from build123d import *

# Parameters (mm, degrees)
SKETCH004_W      = 57.0675
SKETCH004_H      = 36.03
EXTRUDE004_DEPTH = 2
SKETCH005_W      = 57.0675
SKETCH005_H      = 36.03
SKETCH005_R      = 3.5
SKETCH005_R_2    = 2
SKETCH005_W_2    = 9
SKETCH005_H_2    = 3.9474
SKETCH005_W_3    = 4.25
SKETCH005_H_3    = 22
EXTRUDE005_DEPTH = 2


with BuildPart() as obj1:
    # Sketch004 → Extrude004 (new body)
    with BuildSketch(Plane.XY.offset(9)):
        with Locations((15.9391, 12.4324)):
            Rectangle(SKETCH004_W, SKETCH004_H)
        Polygon((-11.59465, 29.4474), (43.47285, 29.4474), (43.47285, -4.5826), (-11.59465, -4.5826), (-11.59465, 5.4324), (-10.59465, 5.4324), (-10.59465, 19.4324), (-11.59465, 19.4324), align=None, mode=Mode.SUBTRACT)
    extrude(amount=EXTRUDE004_DEPTH)


with BuildPart() as tampa002:
    # Sketch005 → Extrude005 (new body)
    with BuildSketch(Plane.XY.offset(11)):
        with Locations((15.9391, 12.4324)):
            Rectangle(SKETCH005_W, SKETCH005_H)
        with Locations((19.3, 18.9)):
            Circle(SKETCH005_R, mode=Mode.SUBTRACT)
        with Locations((28.05086, 23.2)):
            Circle(SKETCH005_R_2, mode=Mode.SUBTRACT)
        with BuildLine():
            ThreePointArc((8.018237, 22.4), (5.85664, 26.85), (3.695043, 22.4))
            Line((3.695043, 22.4), (8.018237, 22.4))
        make_face(mode=Mode.SUBTRACT)
        with Locations((13.75, 25.4737)):
            Rectangle(SKETCH005_W_2, SKETCH005_H_2, mode=Mode.SUBTRACT)
        with Locations((36.375, 12.5)):
            Rectangle(SKETCH005_W_3, SKETCH005_H_3, mode=Mode.SUBTRACT)
        with BuildLine():
            ThreePointArc((11.7, 3.85), (9.2, 1.35), (11.7, -1.15))
            Line((11.7, -1.15), (16.8, -1.15))
            ThreePointArc((16.8, -1.15), (19.3, 1.35), (16.8, 3.85))
            Line((11.7, 3.85), (16.8, 3.85))
        make_face(mode=Mode.SUBTRACT)
    extrude(amount=EXTRUDE005_DEPTH)

    # Fusion001: union obj1
    add(obj1.part)


solid = tampa002.part
Can you work these out from the model? Positions are in its coordinate system, mm. A direction names the side the tool comes from. Round coordinates to 2 decimals unless told otherwise and drop trailing zeros. Order: outer loops, then holes, each group sorted by start corner. A loop starts at its lowest first (then second) coordinate and runs counter-clockwise, first axis right, second up. Notation, with made-up numbers: (64, -16) -> (111, -16) arc R16 ccw to (111, 2) -> close; hole circle Ø6 at (67.5, 6.5). An arc over 180 degrees is marked (long way). Write each question's results on one line, items separated by ' | '. Start each with the question number.
Item 1: Will this pin go through, and if not, where does the flat tip stop? pin 1 (2 mm diameter, centred on x = -5, y = 15.5, fed in from -Z).
Item 2: If we section it at C-C, the plane z = 12.45: Write out the boundary of the cut face in (x, y), then the cut area to 3 significant figures.
Item 3: Which directions (+Z, -Z, +X, -X, +Y, -Y) give clear straight access to the entire face, cutting with the end or side of a thin tool? Please do faces 4 (the flat face through (44.473, 12, 11)), 5 (the flat face through (43.473, 13, 10)), 6 (the flat face through (18.25, 25, 12)).
Item 4: If we section it at A-A, the plane y = 12: Write out the boundary of the cut face in (x, z), then the cut area to 3 significant figures.
Item 5: Please list where these lines run through material, in increasing order: L1, parallel to Y at x = 13, z = 11.8; L2, parallel to X at y = 18, z = 9.7; L3, parallel to Y at x = 18, z = 9.35.
Item 6: If we section it at B-B, the plane z = 9.75: Write out the boundary of the cut face in (x, y).
Item 7: Thinking about a two-plate mould opening in X: for faces 1 (the flat face through (-12.595, 12, 11)), 2 (the flat face through (16, 13, 13)), 3 (the cylindrical face through (5.94, 26.85, 11.99)), which applies, +X half, -X half, draft (parallel to the pull), parting line (faces both ways), or undercut?
Item 8: If we section it at D-D, the plane x = -4: Write out the boundary of the cut face in (y, z).
Results:
1) pin 1: stops at z = 11
2) outline: (-12.59, -5.58) -> (44.47, -5.58) -> (44.47, 30.45) -> (-12.59, 30.45) -> close; hole (3.7, 22.4) -> (8.02, 22.4) arc R2.75 ccw (long way) to start; hole (9.25, 23.5) -> (18.25, 23.5) -> (18.25, 27.45) -> (9.25, 27.45) -> close; hole (11.7, -1.15) -> (16.8, -1.15) arc R2.5 ccw to (16.8, 3.85) -> (11.7, 3.85) arc R2.5 ccw to start; hole circle Ø7 at (19.3, 18.9); hole circle Ø4 at (28.05, 23.2); hole (34.25, 1.5) -> (38.5, 1.5) -> (38.5, 23.5) -> (34.25, 23.5) -> close | area: 1,810 mm2
3) face 4: +Z, -Z, +X, +Y, -Y | face 5: -Z | face 6: +Z, -Z
4) outline: (-12.59, 9) -> (-10.59, 9) -> (-10.59, 11) -> (34.25, 11) -> (34.25, 13) -> (-12.59, 13) -> close; (38.5, 11) -> (43.47, 11) -> (43.47, 9) -> (44.47, 9) -> (44.47, 13) -> (38.5, 13) -> close | area: 112 mm2
5) L1: y = -5.58 to -1.15, 3.85 to 23.5, 27.45 to 30.45 | L2: x = -12.59 to -10.59, 43.47 to 44.47 | L3: y = -5.58 to -4.58, 29.45 to 30.45
6) outline: (-12.59, -5.58) -> (44.47, -5.58) -> (44.47, 30.45) -> (-12.59, 30.45) -> close; hole (-11.59, -4.58) -> (43.47, -4.58) -> (43.47, 29.45) -> (-11.59, 29.45) -> (-11.59, 19.43) -> (-10.59, 19.43) -> (-10.59, 5.43) -> (-11.59, 5.43) -> close
7) face 1: -X half | face 2: draft | face 3: undercut
8) outline: (-5.58, 9) -> (-4.58, 9) -> (-4.58, 11) -> (29.45, 11) -> (29.45, 9) -> (30.45, 9) -> (30.45, 13) -> (-5.58, 13) -> close
